Here's the drawing with two shaded views (mm, measured from the low corner). I have some questions. A direction names the side the tool comes from. Give positions to 0.01 mm unless a question says otherwise; leave off trailing zeros. Write each loop counter-clockwise with the first axis right and the second up, starting at its lowest first coordinate (ties: lowest second). Pieces come first, ordered by that corner, then holes. Notation, with made-up numbers: M -37.75,-9.5 L -31.75,-9.5 A24 cw -31.75,13.5 Z; hole C 5,81.5 d9. An arc over 180 degrees is marked long. Answer as a JSON object with one key per item and string values. Group by question number.
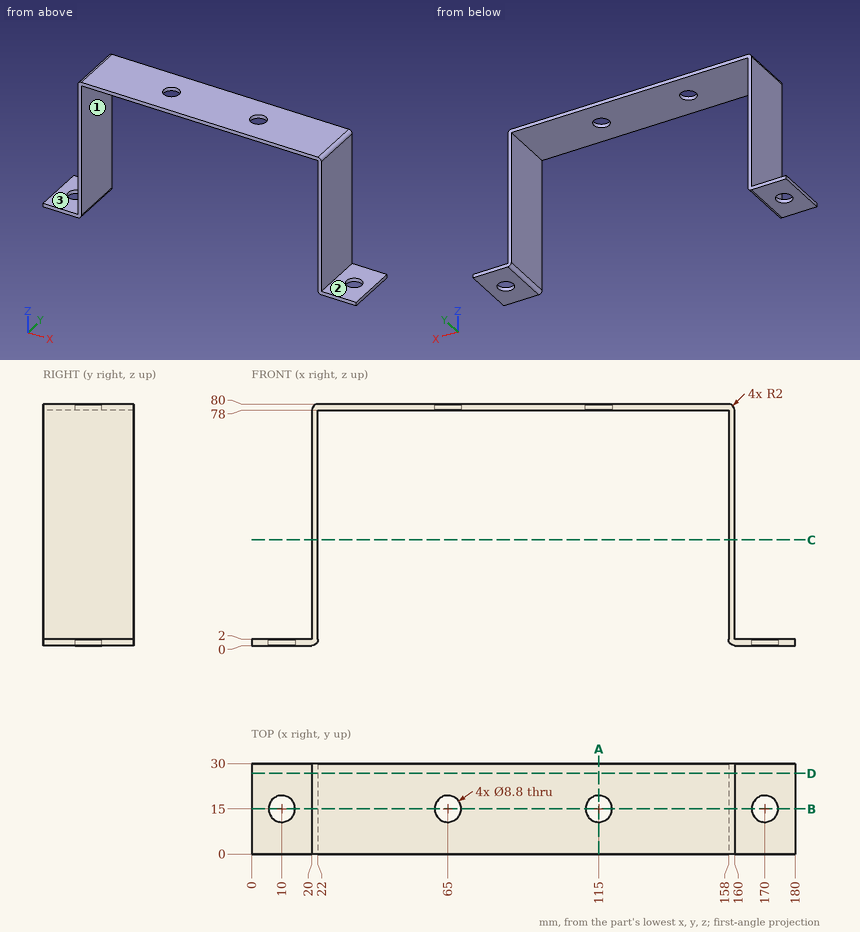
1) Please list where these lines run through material, in increasing order: line 1 along X through (y, z) = (12.25, 25); line 2 along Y through (x, z) = (170, 0.65); line 3 along Z through (x, y) = (127, 7). Write a range as from..to.
2) If we section it at A-A, the plane x = 115: List the corners of the cut face in (y, z) for me.
3) If we section it at D-D, the plane y = 26.75: List the corners of the cut face in (x, z) for me.
4) I'm going to push flat-ended pins straight in: pin 1 (9 mm diameter, centred on x = 78.5, y = 21.5, fed in from -Z); pin 2 (9 mm diameter, centred on y = 18.5, z = 25.5, fed in from -X); pin 3 (15 mm diameter, centred on y = 14.5, z = 25.5, fed in from +X); pin 4 (5.5 mm diameter, centred on x = 170, y = 15, fed in from +Z). Where does each tip first touch, or does it pass through?
5) If we section it at B-B, the plane y = 15: Give the number of separate pieces and of enclosed holes in the cut face, plus the area to 3 significant figures.
6) For the marked faces 1, 2 and 3, which set-ups out of +Z, -Z, +X, -X, +Y, -Y let a thin tool reach every point of the face, with its end or its side?
7) If we section it at C-C, the plane z = 35: List the corners of the cut face in (x, y) for me, plus the area to 3 significant figures.
Taken from the geometry:
{
 "1": {"line 1": "20..22, 158..160", "line 2": "0..10.6, 19.4..30", "line 3": "78..80"},
 "2": {"outline": "M 0,78 L 10.6,78 L 10.6,80 L 0,80 Z; M 19.4,78 L 30,78 L 30,80 L 19.4,80 Z"},
 "3": {"outline": "M 0,0 L 20,0 A2 ccw 22,2 L 22,78 L 158,78 L 158,2 A2 ccw 160,0 L 180,0 L 180,2 L 160,2 L 160,78 A2 ccw 158,80 L 22,80 A2 ccw 20,78 L 20,2 L 0,2 Z"},
 "4": {"pin 1": "z = 78", "pin 2": "x = 20", "pin 3": "x = 160", "pin 4": "through"},
 "5": {"separate pieces": "5", "enclosed holes": "0", "area": "598 mm²"},
 "6": {"face 1": "-Z, +Y, -Y", "face 2": "+Z, +X, +Y, -Y", "face 3": "+Z, -X, +Y, -Y"},
 "7": {"outline": "M 20,0 L 22,0 L 22,30 L 20,30 Z; M 158,0 L 160,0 L 160,30 L 158,30 Z", "area": "120 mm²"}
}
